Check sheet for the drawn part. Datum: minimum x, y, z corner. Units: mm. Give positions to 0.01 mm unless a question says otherwise; leave off trailing zeros. Loops run counter-clockwise (first coordinate to the right, second up) from the corner with the lowest first, then second, coordinate; pieces in that order, holes last. Notation, with made-up numbers: M 15,45 L 24,45 A14 cw 24,72 Z; hole C -12.75,-28.5 d9. An arc over 180 degrees is marked long. Write each question's results on one line, items separated by ' | '. Start each with the question number.
1. Sectioned sample at A-A on y = 29. Record the cut outline in (x, z).
2. Material ranges on line 1 along Y through (x, z) = (54, 2.2); line 2 along X through (y, z) = (34.5, 1.1); line 3 along X through (y, z) = (44, 1.2), recorded low to high.
3. Sectioned sample at C-C on z = 2.55. Record the cut outline in (x, y).
4. Go/stop test with flat-tipped pins: pin 1 (1.5 mm diameter, centred on x = 81, z = 2, fed in from +Y); pin 2 (0.9 mm diameter, centred on x = 128.5, z = 1, fed in from -Y). Record where each tip stops, or that it passes through.
5. Sectioned sample at B-B on x = 117.5. Record the cut outline in (y, z), and give its area (3 significant figures).
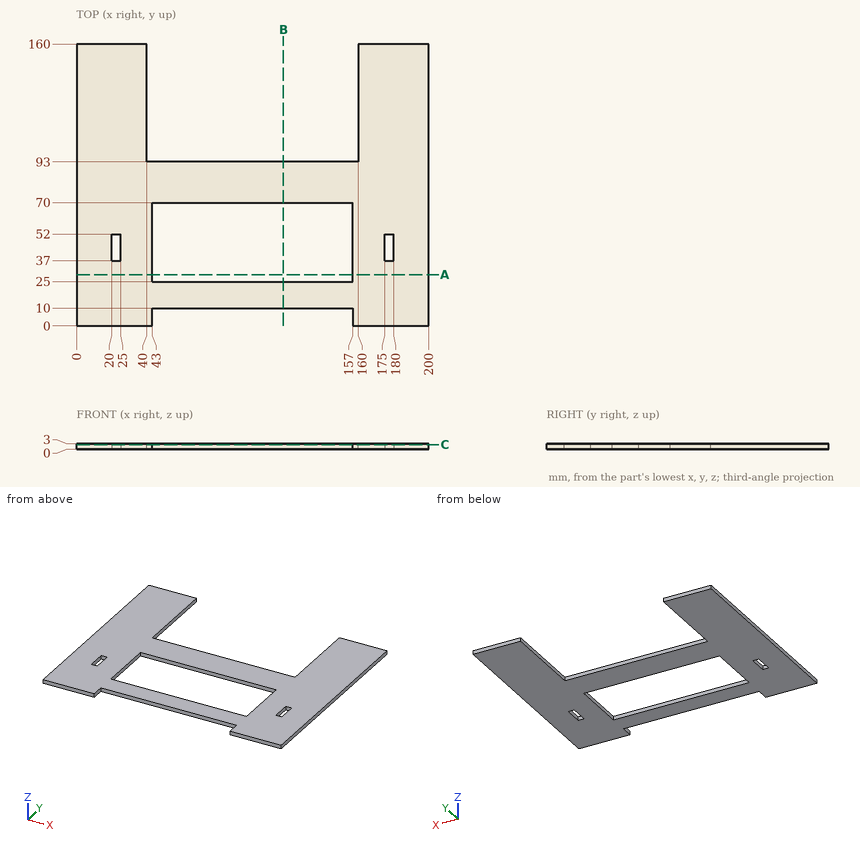
Output values:
1) outline: M 0,0 L 43,0 L 43,3 L 0,3 Z; M 157,0 L 200,0 L 200,3 L 157,3 Z
2) line 1: 10 to 25, 70 to 93 | line 2: 0 to 43, 157 to 200 | line 3: 0 to 20, 25 to 43, 157 to 175, 180 to 200
3) outline: M 0,0 L 43,0 L 43,10 L 157,10 L 157,0 L 200,0 L 200,160 L 160,160 L 160,93 L 40,93 L 40,160 L 0,160 Z; hole M 20,37 L 25,37 L 25,52 L 20,52 Z; hole M 43,25 L 157,25 L 157,70 L 43,70 Z; hole M 175,37 L 180,37 L 180,52 L 175,52 Z
4) pin 1: y = 93 | pin 2: y = 10
5) outline: M 10,0 L 25,0 L 25,3 L 10,3 Z; M 70,0 L 93,0 L 93,3 L 70,3 Z | area: 114 mm2
